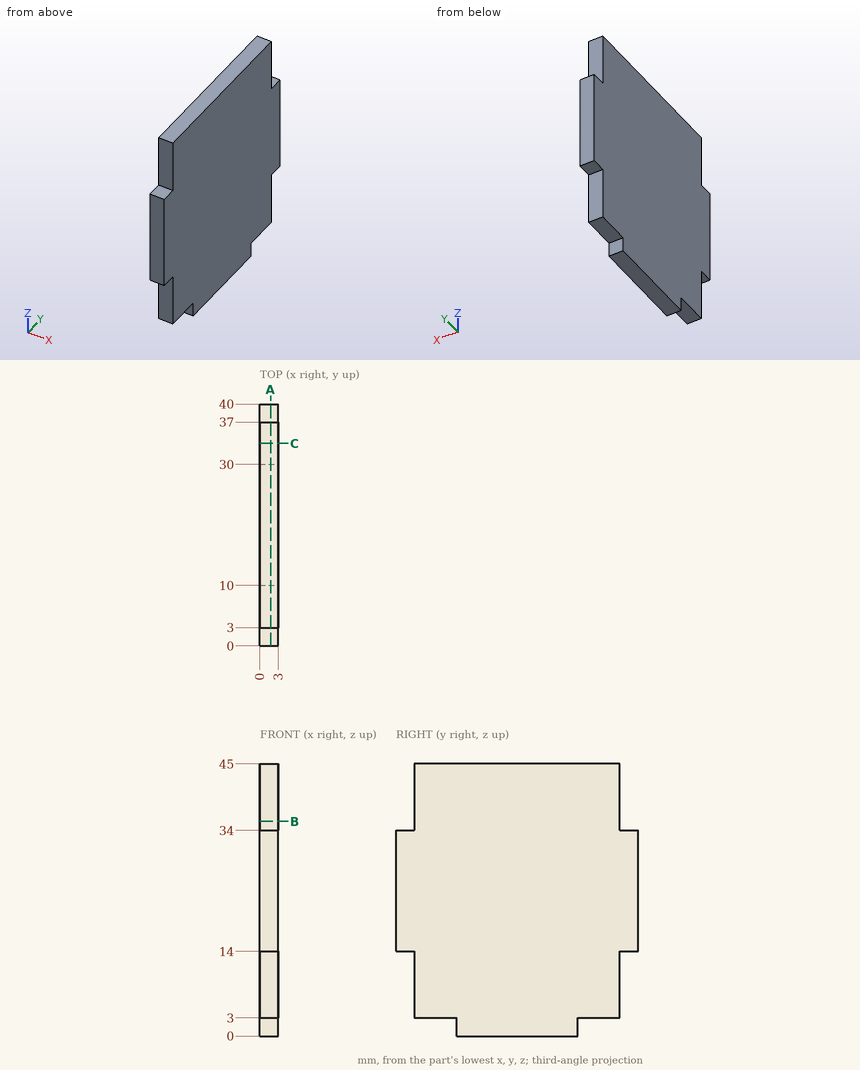
Could you check a few things on this drawing? It's one solid part, dimensions in mm from its lowest x, y, z. Round coordinates to 2 decimals unless told otherwise and drop trailing zeros. Order: outer loops, then holes, each group sorted by start corner. A loop starts at its lowest first (then second) coordinate and runs counter-clockwise, first axis right, second up. Notation, with made-up numbers: M 45.25,62.5 L 89.25,62.5 A20 cw 89.25,74.5 Z; hole C 54,22 d9. An arc over 180 degrees is marked long. Return JSON: item names as keys, results as strings. Group by question number.
1. If we section it at C-C on y = 33.5: List the corners of the cut face in (x, z) for me.
2. If we section it at B-B on z = 35.5: List the corners of the cut face in (x, y) for me, then the cut area to 3 significant figures.
3. Please list where these lines run through material, in increasing order: probe 1 along Y at (x, z) = (1.5, 35); probe 2 along Z at (x, y) = (1.6, 34).
4. If we section it at A-A on x = 1.75: List the corners of the cut face in (y, z) for me, then the cut area to 3 significant figures.
5. I'm going to push flat-ended pins straight in: pin 1 Ø0.9 at (x, z) = (2, 6.5) entering from -Y; pin 2 Ø1.5 at (x, y) = (1.5, 34.5) entering from -Z. Where does each tip first touch, or does it pass through?
Reply:
{
 "1": {"outline": "M 0,3 L 3,3 L 3,45 L 0,45 Z"},
 "2": {"outline": "M 0,3 L 3,3 L 3,37 L 0,37 Z", "area": "102 mm^2"},
 "3": {"probe 1": "3 to 37", "probe 2": "3 to 45"},
 "4": {"outline": "M 0,14 L 3,14 L 3,3 L 10,3 L 10,0 L 30,0 L 30,3 L 37,3 L 37,14 L 40,14 L 40,34 L 37,34 L 37,45 L 3,45 L 3,34 L 0,34 Z", "area": "1,610 mm^2"},
 "5": {"pin 1": "y = 3", "pin 2": "z = 3"}
}
